```python
from build123d import *

# Parameters (mm, degrees)
F1_DEPTH = 1.525
F2_R     = 9
F2_R_2   = 1.535
F2_R_3   = 1.75
F2_R_4   = 2.035
F3_DEPTH = 3.051
F6_DEPTH = 3.05


# Not quite as in the source:
# - a pattern or mirror of a feature is missing from the dataset's text; its kind, count and spacing are read off the source's solid


with BuildPart() as f1:
    # F0 (on Top) → F1 (new body, symmetric)
    with BuildSketch(Plane.XY):
        with BuildLine():
            Line((122, 52.8), (-4.2365988975, 52.8))
            ThreePointArc((-4.2365988975, 52.8), (-12.8402454427, 55.5127193357), (-18.3319882093, 62.6696978501))
            Line((-18.3319882093, 62.6696978501), (-21, 70))
            ThreePointArc((-21, 70), (-32.1803398875, 67.360679775), (-41, 60))
            ThreePointArc((-41, 60), (-55.8683298051, 31.6227766017), (-61, 0))
            Line((-61, 0), (137, 0))
            ThreePointArc((137, 0), (135.6994290201, 19.038602614), (131.8218801501, 37.7234758844))
            ThreePointArc((131.8218801501, 37.7234758844), (128.067905641, 46.0154645332), (122, 52.8))
        make_face()
    extrude(amount=F1_DEPTH, both=True)

    # F2 (on face) → F3 (cut, through all)
    with BuildSketch(Plane.XY.offset(1.525)):
        Circle(F2_R)
        with Locations((-52, 21)):
            Circle(F2_R_2)
        with Locations((-52, 7)):
            Circle(F2_R_2)
        with Locations((-35, 46.5)):
            Circle(F2_R_2)
        with Locations((-20.5, 46.25)):
            Circle(F2_R_2)
        with Locations((-17.5, 27.5)):
            Circle(F2_R_2)
        with Locations((-17.5, 22.25)):
            Circle(F2_R_2)
        with Locations((-10.5, 34.5)):
            Circle(F2_R_3)
        with Locations((-9.5, 23.75)):
            Circle(F2_R_2)
        with Locations((15.75, 0)):
            Circle(F2_R_2)
        with Locations((25.5, 0)):
            Circle(F2_R_2)
        with Locations((47, 34)):
            Circle(F2_R_2)
        with Locations((55, 34)):
            Circle(F2_R_2)
        with Locations((62.5, 24)):
            Circle(F2_R_2)
        with Locations((67, 45)):
            Circle(F2_R_2)
        with Locations((73.5, 27.5)):
            Circle(F2_R_2)
        with Locations((78, 22.5)):
            Circle(F2_R_3)
        with Locations((83.5, 0)):
            Circle(F2_R_2)
        with Locations((94, 0)):
            Circle(F2_R_2)
        with Locations((91, 33.5)):
            Circle(F2_R_3)
        with Locations((89.5, 46.5)):
            Circle(F2_R_2)
        with Locations((98.5, 44.5)):
            Circle(F2_R_2)
        with Locations((103, 15)):
            Circle(F2_R_4)
        with Locations((123, 22.5)):
            Circle(F2_R_2)
        with Locations((127.5, 27)):
            Circle(F2_R_2)
        with Locations((127.5, 15)):
            Circle(F2_R_4)
    extrude(amount=-F3_DEPTH, mode=Mode.SUBTRACT)

    # F4: F1 across face


with BuildPart() as f1_1:
    add(f1.part)
    add(f1.part.mirror(Plane(origin=(54.5, 0, 0), x_dir=(1, 0, 0), z_dir=(0, -1, 0))))

    # F5 (on face) → F6 (cut, through all)
    with BuildSketch(Plane.XY.offset(1.525)):
        Polygon((46, 31), (34, 31), (34, 35.5), (28, 35.5), (28, 31), (16, 31), (16, 26), (28, 26), (28, 21.5), (34, 21.5), (34, 26), (46, 26), align=None)
    f6 = extrude(amount=-F6_DEPTH, mode=Mode.SUBTRACT)

    # F6_copies: F6 across plane
    add(f6.mirror(Plane(origin=(0, 0, 0), x_dir=(0, 0, -1), z_dir=(0, -1, 0))), mode=Mode.SUBTRACT)


solid = f1_1.part
```
For this review, take the finished solid that the model builds, in its own axes (mm). Give positions to 0.01 mm unless a question says otherwise; leave off trailing zeros. Write each loop counter-clockwise with the first axis right and the second up, starting at its lowest first coordinate (ties: lowest second). Pieces come first, ordered by that corner, then holes.
Item 1: Take a section at B-B (z = -0.05). Give the number of separate pieces and of enclosed holes in the cut face, and give its area (3 significant figures).
Item 2: Wall thickness on probe 1 along Y at (x, z) = (47, -0.3) (3 decimals); probe 2 along Y at (x, z) = (67, 0.95) (3 decimals); probe 3 along Y at (x, z) = (127.5, 0.15) (3 decimals): over which ranges is each line inside the solid? List them lowest first.
Item 3: The part is to be moulded in two halves that separate along X. For faces 1 (the face through (-32.035, 67.433, 0.021)), 2 (the face through (128.138, 45.908, 0.021)), 3 (the face through (101.385, 13.762, 0.021)), say which applies: +X half, -X half, draft (parallel to the pull), parting line (faces both ways), or undercut.
Item 4: Insertion check: P1, Ø0.9, axis at y = -32.5, z = 0.5, coming from the -X side; P2, Ø1.5, axis at x = 40.5, z = -0.5, coming from the +Y side. Each pin has a flat end and moves straight along its axis. Give the tip position at first contact, or say it passes through.
Item 5: Take a section at C-C (y = 56). Give the boundary of the cut face in (x, z) (3 decimals).
Item 6: Take a section at A-A (x = 21.5). Give the boundary of the cut face in (y, z) (3 decimals).
Established:
1. separate pieces: 1
1. enclosed holes: 49
1. area: 19,700 mm2
2. probe 1: y = -52.8 to -35.535, -32.465 to 32.465, 35.535 to 52.8
2. probe 2: y = -52.8 to -46.535, -43.465 to 43.465, 46.535 to 52.8
2. probe 3: y = -46.856 to -28.535, -25.465 to -17.035, -12.965 to 12.965, 17.035 to 25.465, 28.535 to 46.856
3. face 1: -X half
3. face 2: +X half
3. face 3: undercut
4. P1: stops at x = -55.72
4. P2: stops at y = 52.8
5. outline: (-43.849, -1.525) - (-13.497, -1.525) - (-13.497, 1.525) - (-43.849, 1.525) - close
6. outline: (-52.8, -1.525) - (-31, -1.525) - (-31, 1.525) - (-52.8, 1.525) - close; (-26, -1.525) - (26, -1.525) - (26, 1.525) - (-26, 1.525) - close; (31, -1.525) - (52.8, -1.525) - (52.8, 1.525) - (31, 1.525) - close
